from build123d import *

# Parameters (mm, degrees)
F0_W     = 139.7
F0_H     = 387.35
F1_DEPTH = 19.05
F2_W     = 22.225
F2_H     = 47.625
F3_DEPTH = 19.051
F6_DEPTH = 19.051


# Not quite as in the source:
# - a length typed as a fraction of an inch, garbled in the dataset ("3 / 203.2 mm" for 3/8 in), is restored
# - a pattern or mirror of a feature is missing from the dataset's text; its kind, count and spacing are read off the source's solid


with BuildPart() as f1:
    # F0 (on Front) → F1 (new body)
    with BuildSketch(Plane.XZ):
        with Locations((69.85, 193.675)):
            Rectangle(F0_W, F0_H)
    extrude(amount=F1_DEPTH)

    # F2 (on face) → F3 (cut, through all)
    with BuildSketch(Plane.XZ.offset(19.05)):
        with Locations((11.1125, 363.5375)):
            Rectangle(F2_W, F2_H)
    f3 = extrude(amount=-F3_DEPTH, mode=Mode.SUBTRACT)

    # F3_copies: F3 across plane
    add(f3.mirror(Plane(origin=(69.85, 0, 0), x_dir=(0, 0, 1), z_dir=(1, 0, 0))), mode=Mode.SUBTRACT)

    # F5 (on face) → F6 (cut, through all)
    with BuildSketch(Plane.XZ.offset(19.05)):
        Polygon((0, 50.8), (0, 0), (19.05, 50.8), align=None)
    f6 = extrude(amount=-F6_DEPTH, mode=Mode.SUBTRACT)

    # F6_copies: F6 across plane
    add(f6.mirror(Plane(origin=(69.85, 0, 0), x_dir=(0, 0, 1), z_dir=(1, 0, 0))), mode=Mode.SUBTRACT)


solid = f1.part
Model file for the job. Use its own axes, mm. A direction names the side the tool comes from. Coordinates: 2 decimals unless noted, no trailing zeros. Order: outer loops, then holes, each group sorted by start corner. A loop starts at its lowest first (then second) coordinate and runs counter-clockwise, first axis right, second up. Notation, with made-up numbers: (-27.5, 86.5) -> (-0.5, 86.5) arc R27 cw to (-0.5, 103.5) -> close; hole circle Ø11 at (8.5, 83). An arc over 180 degrees is marked (long way). Return JSON: item names as keys, results as strings. Group by question number.
Item 1: Saw through at B-B on z = 28. Write the cut outline in (x, y), then the cut area to 3 significant figures.
Item 2: Saw through at A-A on y = -5.25. Write the cut outline in (x, z) (3 decimals).
Item 3: Tool access for faces 1 (the flat face through (130, -10, 50.8)), 2 (the flat face through (22.225, -10, 363)), 3 (the flat face through (69, 0, 196)), 4 (the flat face through (69, -19.05, 196)), 5 (the flat face through (129, -10, 339.725)): list every direction of +Z, -Z, +X, -X, +Y, -Y with a clear straight run to the whole face (end or side of a thin tool).
Item 4: Pull direction Z, two halves, no side cores. Call faces 6 (the flat face through (117.475, -10, 363)), 7 (the flat face through (9.39, -9.66, 25.04)), 8 (the flat face through (69, -9, 387.35)): pulls with the +Z half, pulls with the -Z half, needs draft (parallel to the pull), parting line crosses it, or undercut.
Item 5: Wall check: line 1 along X through (y, z) = (-6, 19) (3 decimals); line 2 along X through (y, z) = (-0.75, 368) (3 decimals). Give the ranges that are in metal, low to high. Write a range as [from, to].
Item 6: Flat gauge pins, fed straight in: P1, Ø5.5, axis at y = -7, z = 372.5, coming from the -X side (3 decimals); P2, Ø9.5, axis at y = -12.5, z = 354.5, coming from the +X side (3 decimals); P3, Ø5.5, axis at x = 124, y = -10, coming from the +Z side (3 decimals). Where does each tip first touch, or does it go through?
Values found:
{
 "1": {"outline": "(10.5, -19.05) -> (129.2, -19.05) -> (129.2, 0) -> (10.5, 0) -> close", "area": "2,260 mm2"},
 "2": {"outline": "(0, 0) -> (139.7, 0) -> (120.65, 50.8) -> (139.7, 50.8) -> (139.7, 339.725) -> (117.475, 339.725) -> (117.475, 387.35) -> (22.225, 387.35) -> (22.225, 339.725) -> (0, 339.725) -> (0, 50.8) -> (19.05, 50.8) -> close"},
 "3": {"face 1": "+X, +Y, -Y", "face 2": "+Z, -X, +Y, -Y", "face 3": "+Z, -Z, +X, -X, +Y", "face 4": "+Z, -Z, +X, -X, -Y", "face 5": "+Z, +X, +Y, -Y"},
 "4": {"face 6": "needs draft", "face 7": "undercut", "face 8": "pulls with the +Z half"},
 "5": {"line 1": "x = [7.125, 132.575]", "line 2": "x = [22.225, 117.475]"},
 "6": {"P1": "stops at x = 22.225", "P2": "stops at x = 117.475", "P3": "stops at z = 339.725"}
}
